```python
from build123d import *

# Parameters (mm, degrees)
F1_DEPTH = 3


with BuildPart() as f1:
    # F0 (on Front) → F1 (new body)
    with BuildSketch(Plane.XZ):
        Polygon((-42.78, 0), (-39.78, 0), (-39.78, 3.02), (-36.74, 3.02), (-36.74, 0), (-1.52, 0), (-1.52, 3.02), (1.52, 3.02), (1.52, 0), (36.74, 0), (36.74, 3.02), (39.78, 3.02), (39.78, 0), (42.78, 0), (42.78, 12), (39.78, 12), (39.78, 8.98), (36.74, 8.98), (36.74, 12), (1.52, 12), (1.52, 8.98), (-1.52, 8.98), (-1.52, 12), (-36.74, 12), (-36.74, 8.98), (-39.78, 8.98), (-39.78, 12), (-42.78, 12), align=None)
    extrude(amount=F1_DEPTH)


solid = f1.part
```
The listing builds one solid part. Answer for the finished solid, in the listing's coordinates (mm). A direction names the side the tool comes from. Give positions to 0.01 mm unless a question says otherwise; leave off trailing zeros. Order: outer loops, then holes, each group sorted by start corner. A loop starts at its lowest first (then second) coordinate and runs counter-clockwise, first axis right, second up. Notation, with made-up numbers: (82.5, 34.5) -> (139.5, 34.5) arc R17 ccw to (139.5, 39.5) -> close; hole circle Ø6 at (28, -12). An arc over 180 degrees is marked (long way). Write each question's results on one line, items separated by ' | '.
Q1. The part is cut by section A-A, the plane z = 1. Give the vertices of the cut face in (x, y).
Checked values:
outline: (-42.78, -3) -> (-39.78, -3) -> (-39.78, 0) -> (-42.78, 0) -> close; (-36.74, -3) -> (-1.52, -3) -> (-1.52, 0) -> (-36.74, 0) -> close; (1.52, -3) -> (36.74, -3) -> (36.74, 0) -> (1.52, 0) -> close; (39.78, -3) -> (42.78, -3) -> (42.78, 0) -> (39.78, 0) -> close
Q2. Which of the six approach directions +Z, -Z, +X, -X, +Y, -Y give full straight-line access (tool end or side, diameter ignored) to faces 1 (the face through (-19, -1, 12)), 2 (the face through (36.74, -1, 1)), 3 (the face through (-1.52, -1, 10))?
Checked values:
face 1: +Z, +X, -X, +Y, -Y | face 2: -Z, +Y, -Y | face 3: +Z, +Y, -Y
Q3. The part is cut by section B-B, the plane y = -1.9. Give the vertices of the cut face in (x, z), and give its area (3 significant figures).
Checked values:
outline: (-42.78, 0) -> (-39.78, 0) -> (-39.78, 3.02) -> (-36.74, 3.02) -> (-36.74, 0) -> (-1.52, 0) -> (-1.52, 3.02) -> (1.52, 3.02) -> (1.52, 0) -> (36.74, 0) -> (36.74, 3.02) -> (39.78, 3.02) -> (39.78, 0) -> (42.78, 0) -> (42.78, 12) -> (39.78, 12) -> (39.78, 8.98) -> (36.74, 8.98) -> (36.74, 12) -> (1.52, 12) -> (1.52, 8.98) -> (-1.52, 8.98) -> (-1.52, 12) -> (-36.74, 12) -> (-36.74, 8.98) -> (-39.78, 8.98) -> (-39.78, 12) -> (-42.78, 12) -> close | area: 972 mm^2
Q4. Each of these flat-tipped pins is pushed along its axis until it touches: P1, Ø1.5, axis at x = 6.5, z = 2, coming from the +Y side; P2, Ø0.9, axis at x = 38, y = -1, coming from the -Z side. Where does it stop, or does it pass through?
Checked values:
P1: stops at y = 0 | P2: stops at z = 3.02
Q5. Straight lines are drawn through the part: probe 1 along X at (y, z) = (-1.65, 10.5); probe 2 along Z at (x, y) = (0, -2.55). For each, find the intervals that lie inside material, in ascending order. Write a range as from..to.
Checked values:
probe 1: x = -42.78..-39.78, -36.74..-1.52, 1.52..36.74, 39.78..42.78 | probe 2: z = 3.02..8.98
Q6. Determine the mould class of faces 4 (the face through (19, -1, 12)), 5 (the face through (0, -1, 3.02)), 6 (the face through (39.78, -1, 11)) for opening direction X: pulls with the +X half, pulls with the -X half, needs draft (parallel to the pull), parting line crosses it, or undercut.
Checked values:
face 4: needs draft | face 5: undercut | face 6: undercut
